from build123d import *

# Parameters (mm, degrees)
F0_R     = 12.7
F1_DEPTH = 1.524
F2_R     = 13.97
F3_DEPTH = 0.762
F4_W     = 5.08
F4_H     = 1.524
F6_W     = 5.08000508
F6_H     = 1.5265774739
F7_DEPTH = 0.254
F8_R     = 0.25399


# Not quite as in the source:
# - a fillet or chamfer is up to 0.001 mm smaller than in the source, because OpenCascade refuses the exact size


with BuildPart() as f1:
    # F0 (on Top) → F1 (new body)
    with BuildSketch(Plane.XY):
        Circle(F0_R)
    extrude(amount=F1_DEPTH)

    # F2 (on Top) → F3 (join)
    with BuildSketch(Plane.XY):
        Circle(F2_R)
    extrude(amount=F3_DEPTH)

    # F4 (on Front) → F5 (revolve, cut)
    with BuildSketch(Plane.XZ):
        Rectangle(F4_W, F4_H)
    revolve(axis=Axis((0, 0, -0.762), (-1, 0, 0)), mode=Mode.SUBTRACT)

    # F6 (on Top) → F7 (join)
    with BuildSketch(Plane.XY):
        Rectangle(F6_W, F6_H)
    extrude(amount=F7_DEPTH)

    # F8 (radius 0.254 in the source; OpenCascade refuses exactly that, so slightly less here)
    f8_edges = [f1.edges().sort_by_distance(p)[0] for p in [
        (0, 0.763289, 0.254),
        (0, -0.763289, 0.254),
    ]]
    fillet(f8_edges, radius=F8_R)


solid = f1.part
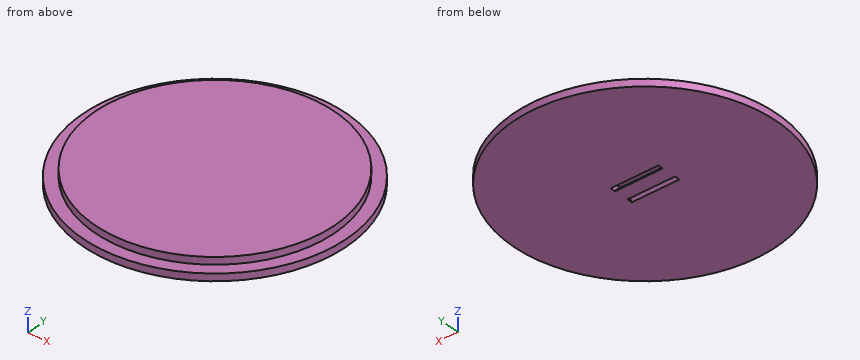
The model under review builds one solid part; all positions refer to its coordinate system, in mm. Give positions to 0.01 mm unless a question says otherwise; leave off trailing zeros. Write each loop counter-clockwise with the first axis right and the second up, starting at its lowest first coordinate (ties: lowest second). Pieces come first, ordered by that corner, then holes. Notation, with made-up numbers: M -19,11 L -4,11 A16 cw -4,21 Z; hole C 33,61.5 d5. An arc over 180 degrees is marked long. One line per question, with ' | ' between items. Start each with the question number.
Item 1: We need section C-C on z = 1.1. Write out the cut boundary in (x, y).
Item 2: We need section A-A on y = 0. Write out the cut boundary in (x, z), plus the area to 3 significant figures.
Item 3: We need section D-D on y = 10.25. Write out the cut boundary in (x, z).
Item 4: Wall thickness on line 1 (X direction, y = 0.25, z = 0.35); line 2 (Y direction, x = -0.25, z = 1.3); line 3 (X direction, y = 5.25, z = 1.05): over which ranges is each line inside the solid? List them lowest first. Write a range as from..to.
Results found:
1) outline: C 0,0 d25.4
2) outline: M -13.97,0 L 13.97,0 L 13.97,0.76 L 12.7,0.76 L 12.7,1.52 L -12.7,1.52 L -12.7,0.76 L -13.97,0.76 Z; hole M -2.54,0.25 L 2.54,0.25 L 2.54,0.76 L -2.54,0.76 Z | area: 38.1 mm2
3) outline: M -9.49,0 L 9.49,0 L 9.49,0.76 L 7.5,0.76 L 7.5,1.52 L -7.5,1.52 L -7.5,0.76 L -9.49,0.76 Z
4) line 1: x = -13.97..-2.54, 2.54..13.97 | line 2: y = -12.7..12.7 | line 3: x = -11.56..11.56
